```python
from build123d import *

# Parameters (mm, degrees)
F0_W     = 119.039789
F0_H     = 64.663587
F1_DEPTH = 25.4
F2_R     = 5.08
F3_R     = 5.08


with BuildPart() as f1:
    # F0 (on Front) → F1 (new body)
    with BuildSketch(Plane.XZ):
        with Locations((-1.224685, -2.204438)):
            Rectangle(F0_W, F0_H)
    extrude(amount=F1_DEPTH)

    # F2
    f2_edges = [f1.edges().sort_by_distance(p)[0] for p in [
        (58.295209, -12.7, 30.127356),
        (58.295209, -12.7, -34.536231),
        (-60.74458, -12.7, 30.127356),
        (-60.74458, -12.7, -34.536231),
    ]]
    fillet(f2_edges, radius=F2_R)

    # F3
    f3_edges = [f1.edges().sort_by_distance(p)[0] for p in [
        (-60.74458, -25.4, -2.204438),
        (-60.74458, 0, -2.204438),
    ]]
    fillet(f3_edges, radius=F3_R)


solid = f1.part
```
For this review, take the finished solid that the model builds, in its own axes (mm). Coordinates: 2 decimals unless noted, no trailing zeros. Loops run counter-clockwise (first coordinate to the right, second up) from the corner with the lowest first, then second, coordinate; pieces in that order, holes last. Notation, with made-up numbers: (-26.75, 26) -> (-4.75, 26) arc R10 ccw to (-4.75, 45) -> close; hole circle Ø6 at (12.25, 67.5). An arc over 180 degrees is marked (long way). Return JSON: item names as keys, results as strings. Group by question number.
(1) To check wall thickness, follow L1, parallel to X at y = -4.75, z = -22; L2, parallel to Z at x = 43.5, y = -20.75; L3, parallel to Z at x = -14, y = -2.5. State the ranges of each line that lie inside material, in increasing order.
(2) For pin 1 Ø1.5 at (x, y) = (-43.5, -22) entering from -Z, flat-tipped, find the tip position at first contact; note if it passes through.
(3) Consider section A-A, the plane y = -2.25. Give the boundary of the cut face in (x, z), plus the area to 3 significant figures.
Results below:
{
 "1": {"L1": "x = -60.73 to 58.28", "L2": "z = -34.52 to 30.11", "L3": "z = -33.83 to 29.42"},
 "2": {"pin 1": "stops at z = -34.45"},
 "3": {"outline": "(-59.88, -29.46) arc R4.22 ccw to (-55.66, -33.67) -> (53.22, -33.67) arc R4.22 ccw to (57.43, -29.46) -> (57.43, 25.05) arc R4.22 ccw to (53.22, 29.27) -> (-55.66, 29.27) arc R4.22 ccw to (-59.88, 25.05) -> close", "area": "7,370 mm2"}
}
